```python
from build123d import *

# Parameters (mm, degrees)
F1_DEPTH = 25.4
F2_R     = 31.75
F3_DEPTH = 25.4
F2_R_2   = 3.175
F5_DEPTH = 12.7
F6_DEPTH = 50.8


with BuildPart() as f1:
    # F0 (on Front) → F1 (new body)
    with BuildSketch(Plane.XZ):
        with BuildLine():
            ThreePointArc((27.7778723818, 19.05), (7.2048117222, 54.3824802414), (-30.6421276182, 69.85))
            Line((-30.6421276182, 69.85), (-30.6421276182, -69.85))
            Line((-30.6421276182, -69.85), (27.7778723818, -69.85))
            Line((27.7778723818, -69.85), (27.7778723818, 19.05))
        make_face()
    extrude(amount=F1_DEPTH)

    # F2 (on face) → F3, piece 2 (join)
    with BuildSketch(Plane(origin=(0, 0, -69.85), x_dir=(1, 0, 0), z_dir=(0, 0, -1))):
        with Locations((0, 14.7020313889)):
            Circle(F2_R_2)
    extrude(amount=F3_DEPTH)

    # F5 (cut): a face of the model
    f5_faces = [f1.faces().sort_by_distance(p)[0] for p in [
        (0, -14.7020313889, -95.25),
    ]]
    extrude(f5_faces, amount=-F5_DEPTH, mode=Mode.SUBTRACT)

    # F6 (cut): a face of the model
    f6_faces = [f1.faces().sort_by_distance(p)[0] for p in [
        (0, -14.7020313889, -82.55),
    ]]
    extrude(f6_faces, amount=-F6_DEPTH, mode=Mode.SUBTRACT)


with BuildPart() as f3:
    # F2 (on face) → F3 (new body)
    with BuildSketch(Plane(origin=(0, 0, -69.85), x_dir=(1, 0, 0), z_dir=(0, 0, -1))):
        with Locations((0, 116.4425893424)):
            Circle(F2_R)
    extrude(amount=F3_DEPTH)


solid = f1.part
```
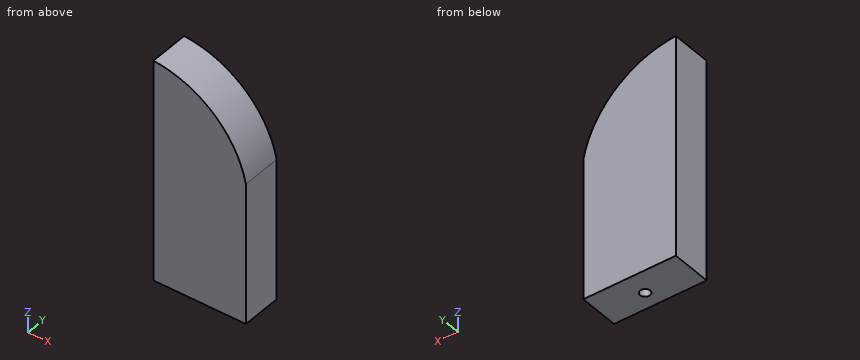
For this review, take the finished solid that the model builds, in its own axes (mm). Coordinates: 2 decimals unless noted, no trailing zeros. Write each loop counter-clockwise with the first axis right and the second up, starting at its lowest first coordinate (ties: lowest second). Pieces come first, ordered by that corner, then holes. Notation, with made-up numbers: (-21, 21.25) - (12, 21.25) arc R30 ccw to (12, 54.25) - close; hole circle Ø8 at (31.5, 2.5). An arc over 180 degrees is marked (long way). Answer in a Markdown table with one row per item. Add a question column.
Q1. For probe 1 along Y at (x, z) = (0, -50.5); probe 2 along X at (y, z) = (-16.5, -44); probe 3 along Z at (x, y) = (-18.5, -13), list the stretches that pass through material, from the lowest coordinate up.
Q2. We need section A-A, the plane x = 0.5. State the section outline as (y, z) points, and give its area (3 significant figures).
Q3. We need section C-C, the plane z = 36.5. State the section outline as (x, y) points.
Q4. We need section B-B, the plane y = -7.25. State the section outline as (x, z) points.
Answer list:
| question | item | result |
|---|---|---|
| 1 | probe 1 | y = -25.4 to -17.88, -11.53 to 0 |
| 1 | probe 2 | x = -30.64 to -2.62, 2.62 to 27.78 |
| 1 | probe 3 | z = -69.85 to 67.93 |
| 2 | outline | (-25.4, -69.85) - (-17.84, -69.85) - (-17.84, -31.75) - (-11.57, -31.75) - (-11.57, -69.85) - (0, -69.85) - (0, 59.47) - (-25.4, 59.47) - close |
| 2 | area | 3,050 mm2 |
| 3 | outline | (-30.64, -25.4) - (21.49, -25.4) - (21.49, 0) - (-30.64, 0) - close |
| 4 | outline | (-30.64, -69.85) - (27.78, -69.85) - (27.78, 19.05) arc R63.5 ccw to (-30.64, 69.85) - close |
